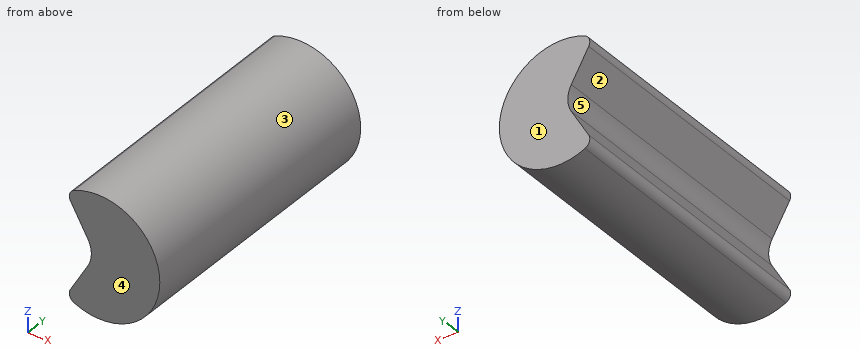
```python
from build123d import *

# Parameters (mm, degrees)
BOSS_EXTRUDE1_DEPTH = 330


with BuildPart() as part:
    # Sketch1 → Boss-Extrude1 (new body)
    with BuildSketch(Plane(origin=(0, 0, 0), x_dir=(1, 0, 0), z_dir=(0, 1, 0))):
        with BuildLine():
            Line((-13.95369343, 15.875), (-35.055377431, 52.424188815))
            ThreePointArc((-35.055377431, 52.424188815), (-35.924016074, 60.457372666), (-30.571566968, 66.51029464))
            ThreePointArc((-30.571566968, 66.51029464), (73.2, 0), (-30.571566968, -66.51029464))
            ThreePointArc((-30.571566968, -66.51029464), (-35.924016074, -60.457372666), (-35.055377431, -52.424188815))
            Line((-35.055377431, -52.424188815), (-13.95369343, -15.875))
            ThreePointArc((-13.95369343, -15.875), (-9.7, 0), (-13.95369343, 15.875))
        make_face()
    extrude(amount=BOSS_EXTRUDE1_DEPTH)


solid = part.part
```
The model under review builds one solid part; all positions refer to its coordinate system, in mm. Face numbers are marked on the shaded views. A direction names the side the tool comes from. Round coordinates to 2 decimals unless told otherwise and drop trailing zeros. Write each loop counter-clockwise with the first axis right and the second up, starting at its lowest first coordinate (ties: lowest second). Pieces come first, ordered by that corner, then holes. Notation, with made-up numbers: (34.25, 50.5) - (88.25, 50.5) arc R6 cw to (88.25, 58.5) - close; hole circle Ø11 at (74.25, -26). An arc over 180 degrees is marked (long way). Answer as CSV lines item,"result". Start each with the question number.
(1) We need section D-D on x = 19.5. State the section outline as (y, z) points.
(2) For the marked faces 1 and 2, list the 3-axis set-ups (+Z, -Z, +X, -X, +Y, -Y) from which the entire face can be reached by the end or side of a thin tool; tool diameter is ignored.
(3) For pin 1 Ø5 at (y, z) = (210, -38.5) entering from +X; pin 2 Ø4 at (y, z) = (171, -30) entering from -X; pin 3 Ø1 at (y, z) = (146.5, 0) entering from -X, all flat-tipped, find the tip position at first contact; note any pin that passes through.
(4) To check wall thickness, follow line 1 (Z direction, x = -20, y = 87.5); line 2 (Z direction, x = 20, y = 133); line 3 (X direction, y = 288, z = -6.5). State the ranges of each line that lie inside material, in increasing order.
(5) Draft analysis for pull direction Z (two halves, no side actions). For the marked faces 3, 4 and 5, state which applies: pulls with the +Z half, pulls with the -Z half, needs draft (parallel to the pull), parting line crosses it, or undercut.
(6) We need section C-C on z = 0. State the section outline as (x, y) points, plus the area to 3 significant figures.
(7) We need section B-B on y = 58. State the section outline as (x, z) points (3 decimals), plus the area to 3 significant figures.
(8) We need section A-A on x = -26. State the section outline as (y, z) points.
Worked answers:
1,outline,"(0, -70.55) - (330, -70.55) - (330, 70.55) - (0, 70.55) - close"
2,face 1,"+Z, -Z, +X, -X, +Y"
2,face 2,"-X, +Y, -Y"
3,pin 1,"x = 63.74"
3,pin 2,"x = -23.26"
3,pin 3,"x = -9.7"
4,line 1,"-70.41 to -26.35, 26.35 to 70.41"
4,line 2,"-70.41 to 70.41"
4,line 3,"-10.37 to 72.91"
5,face 3,"parting line crosses it"
5,face 4,"needs draft"
5,face 5,"undercut"
6,outline,"(-9.7, 0) - (73.2, 0) - (73.2, 330) - (-9.7, 330) - close"
6,area,"27,400 mm²"
7,outline,"(-35.055, -52.424) arc R10 ccw to (-30.572, -66.51) arc R73.2 ccw (long way) to (-30.572, 66.51) arc R10 ccw to (-35.055, 52.424) - (-13.954, 15.875) arc R31.75 cw to (-13.954, -15.875) - close"
7,area,"11,800 mm²"
8,outline,"(0, -68.43) - (330, -68.43) - (330, -36.74) - (0, -36.74) - close; (0, 36.74) - (330, 36.74) - (330, 68.43) - (0, 68.43) - close"
